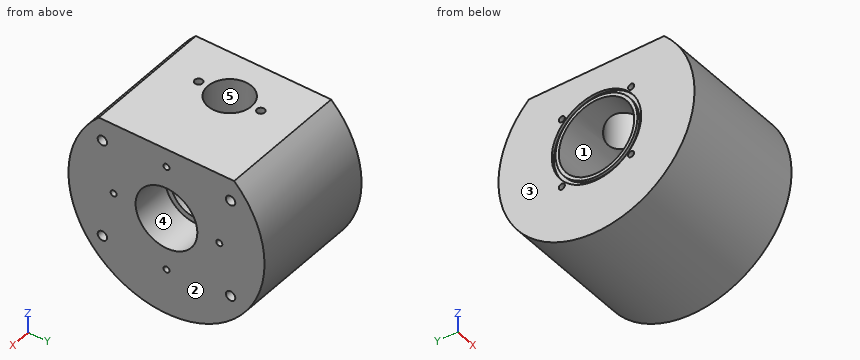
```python
from build123d import *

# Parameters (mm, degrees)
F1_DEPTH  = 106.1974
F2_R      = 25.9969
F3_DEPTH  = 29.9974
F4_R      = 31.75
F5_DEPTH  = 63.5
F6_R      = 17.4625
F7_DEPTH  = 76.201
F8_R      = 21.43125
F8_R_2    = 17.4625
F9_DEPTH  = 7.9248
F10_R     = 18.3769
F11_DEPTH = 33.8506424127
F12_DEPTH = 3.175
F14_D     = 6.5278
F14_DEPTH = 25.4
F14_TIP   = 1.9611489744
F17_D     = 5.1054
F17_DEPTH = 19.05
F17_TIP   = 1.5338169022
F18_R     = 37.6555
F18_R_2   = 34.4805
F19_DEPTH = 2.3622
F20_D     = 5.1054
F20_DEPTH = 19.05
F20_TIP   = 1.5338169022
F22_D     = 7.9375
F22_DEPTH = 25.4
F22_TIP   = 2.3846655818


with BuildPart() as f1:
    # F0 (on Right) → F1 (new body)
    with BuildSketch(Plane.YZ):
        with BuildLine():
            Line((56.9696350292, 59.7408), (-56.9696350292, 59.7408))
            ThreePointArc((-56.9696350292, 59.7408), (0, -82.55), (56.9696350292, 59.7408))
        make_face()
    extrude(amount=-F1_DEPTH)

    # F2 (on face) → F3 (cut)
    with BuildSketch(Plane.YZ):
        Circle(F2_R)
    extrude(amount=-F3_DEPTH, mode=Mode.SUBTRACT)

    # F4 (on face) → F5 (cut)
    with BuildSketch(Plane(origin=(-106.1974, 0, 0), x_dir=(0, -1, 0), z_dir=(-1, 0, 0))):
        Circle(F4_R)
    extrude(amount=-F5_DEPTH, mode=Mode.SUBTRACT)

    # F6 (on face) → F7 (cut, through all)
    with BuildSketch(Plane.YZ.offset(-29.9974)):
        Circle(F6_R)
    extrude(amount=-F7_DEPTH, mode=Mode.SUBTRACT)

    # F8 (on face) → F9 (cut)
    with BuildSketch(Plane.YZ.offset(-29.9974)):
        Circle(F8_R)
        Circle(F8_R_2, mode=Mode.SUBTRACT)
        Circle(F8_R_2)
    extrude(amount=-F9_DEPTH, mode=Mode.SUBTRACT)

    # F10 (on face) → F11 (cut, through all)
    with BuildSketch(Plane.XY.offset(59.7408)):
        with Locations((-68.0974, 0)):
            Circle(F10_R)
    extrude(amount=-F11_DEPTH, mode=Mode.SUBTRACT)

    # F12 (add): a face of the model
    f12_faces = [f1.faces().sort_by_distance(p)[0] for p in [
        (0, 0, 57.5612431238),
    ]]
    extrude(f12_faces, amount=F12_DEPTH)

    # F14
    with Locations(Plane.XY.offset(59.7408)):
        with Locations((-68.0974, 26.1874), (-68.0974, -26.1874)):
            Hole(F14_D / 2, depth=F14_DEPTH)
            with Locations((0, 0, -(F14_DEPTH + F14_TIP / 2))):  # 118° drill point
                Cone(0, F14_D / 2, F14_TIP, mode=Mode.SUBTRACT)

    # F17
    with Locations(Plane.YZ.offset(3.175)):
        with Locations((44.45, 0), (0, -44.45), (-44.45, 0), (0, 44.45)):
            Hole(F17_D / 2, depth=F17_DEPTH)
            with Locations((0, 0, -(F17_DEPTH + F17_TIP / 2))):  # 118° drill point
                Cone(0, F17_D / 2, F17_TIP, mode=Mode.SUBTRACT)

    # F18 (on face) → F19 (cut)
    with BuildSketch(Plane(origin=(-106.1974, 0, 0), x_dir=(0, -1, 0), z_dir=(-1, 0, 0))):
        Circle(F18_R)
        Circle(F18_R_2, mode=Mode.SUBTRACT)
    extrude(amount=-F19_DEPTH, mode=Mode.SUBTRACT)

    # F20
    with Locations(Plane(origin=(-106.1974, 0, 0), x_dir=(0, -1, 0), z_dir=(-1, 0, 0))):
        with Locations((-29.1858323935, 29.1858323935), (29.1858323935, 29.1858323935), (29.1858323935, -29.1858323935), (-29.1858323935, -29.1858323935)):
            Hole(F20_D / 2, depth=F20_DEPTH)
            with Locations((0, 0, -(F20_DEPTH + F20_TIP / 2))):  # 118° drill point
                Cone(0, F20_D / 2, F20_TIP, mode=Mode.SUBTRACT)

    # F22
    with Locations(Plane.YZ.offset(3.175)):
        with Locations((53.975, 41.275), (-53.975, 41.275), (-53.975, -41.275), (53.975, -41.275)):
            Hole(F22_D / 2, depth=F22_DEPTH)
            with Locations((0, 0, -(F22_DEPTH + F22_TIP / 2))):  # 118° drill point
                Cone(0, F22_D / 2, F22_TIP, mode=Mode.SUBTRACT)


solid = f1.part
```
Could you check a few things on this model? Use its own coordinates, in mm. Face numbers are marked on the shaded views. A direction names the side the tool comes from. Give positions to 0.01 mm unless a question says otherwise; leave off trailing zeros. Write each loop counter-clockwise with the first axis right and the second up, starting at its lowest first coordinate (ties: lowest second). Pieces come first, ordered by that corner, then holes. Notation, with made-up numbers: (13.5, 84.25) - (43.5, 84.25) arc R24 cw to (43.5, 105.25) - close; hole circle Ø9 at (88, -7). An arc over 180 degrees is marked (long way). One line per item, written item: value. Start each with the question number.
Item 1: Imagine slicing it at C-C, the plane x = -91. List the corners of the cut face in (y, z) for me.
Item 2: Imagine slicing it at A-A, the plane z = -15.5. List the corners of the cut face in (x, y) for me (3 decimals), and give its area (3 significant figures).
Item 3: If we mould it in two halves opening along X, with no side actions, what happens to the marked faces 3, 4 and 5? For each: +X half, -X half, draft (parallel to the pull), parting line (faces both ways), or undercut.
Item 4: Please list where these lines run through material, in increasing order: line 1 (X direction, y = -19.5, z = -21) (3 decimals); line 2 (Z direction, x = -33, y = 19.5); line 3 (Y direction, x = -16.5, z = 12.5). Write a range as from..to.
Item 5: Which directions (+Z, -Z, +X, -X, +Y, -Y) give clear straight access to the entire face, cutting with the end or side of a thin tool? Please do the marked faces 1 and 2.
Item 6: Imagine slicing it at B-B, the plane y = 15. Give the number of separate pieces and of enclosed holes in the cut face, and give its area (3 significant figures).
Item 7: Imagine slicing it at D-D, the plane z = 6. List the corners of the cut face in (x, y) for me (3 decimals).
Item 8: I'm going to push flat-ended pins straight in: pin 1 (3 mm diameter, centred on y = 44.45, z = 0, fed in from +X); pin 2 (10 mm diameter, centred on y = -20, z = -15.5, fed in from -X); pin 3 (5 mm diameter, centred on y = 53.975, z = -41.275, fed in from +X); pin 4 (8 mm diameter, centred on y = -59.5, z = -65.5, fed in from +X). Where does each tip first touch, or does it pass through?
Geometry says:
1. outline: (-56.97, 59.74) arc R82.55 ccw (long way) to (56.97, 59.74) - close; hole circle Ø63.5 at (0, 0); hole circle Ø5.11 at (-29.19, -29.19); hole circle Ø5.11 at (-29.19, 29.19); hole circle Ø5.11 at (29.19, -29.19); hole circle Ø5.11 at (29.19, 29.19)
2. outline: (-106.197, -81.082) - (3.175, -81.082) - (3.175, -20.871) - (-29.997, -20.871) - (-29.997, -14.8) - (-37.922, -14.8) - (-37.922, -8.043) - (-42.697, -8.043) - (-42.697, -27.709) - (-106.197, -27.709) - (-106.197, -30.8) - (-103.835, -30.8) - (-103.835, -34.317) - (-106.197, -34.317) - close; (-106.197, 27.709) - (-42.697, 27.709) - (-42.697, 8.043) - (-37.922, 8.043) - (-37.922, 14.8) - (-29.997, 14.8) - (-29.997, 20.871) - (3.175, 20.871) - (3.175, 81.082) - (-106.197, 81.082) - (-106.197, 34.317) - (-103.835, 34.317) - (-103.835, 30.8) - (-106.197, 30.8) - close
2. area: 12,500 mm^2
3. face 3: -X half
3. face 4: draft
3. face 5: undercut
4. line 1: -42.697..3.175
4. line 2: -80.21..-8.89, 8.89..59.74
4. line 3: -81.6..-22.79, 22.79..81.6
5. face 1: -X
5. face 2: +Z, -Z, +X, +Y, -Y
6. separate pieces: 3
6. enclosed holes: 0
6. area: 9,430 mm^2
7. outline: (-106.197, -82.332) - (3.175, -82.332) - (3.175, -25.295) - (-29.997, -25.295) - (-29.997, -20.574) - (-37.922, -20.574) - (-37.922, -16.399) - (-42.697, -16.399) - (-42.697, -31.178) - (-106.197, -31.178) - (-106.197, -33.954) - (-103.835, -33.954) - (-103.835, -37.174) - (-106.197, -37.174) - close; (-106.197, 31.178) - (-42.697, 31.178) - (-42.697, 16.399) - (-37.922, 16.399) - (-37.922, 20.574) - (-29.997, 20.574) - (-29.997, 25.295) - (3.175, 25.295) - (3.175, 82.332) - (-106.197, 82.332) - (-106.197, 37.174) - (-103.835, 37.174) - (-103.835, 33.954) - (-106.197, 33.954) - close
8. pin 1: x = -16.51
8. pin 2: x = -42.7
8. pin 3: x = -23.11
8. pin 4: through
